Design review of the part built by this model. Coordinates are the model's own, in mm. Coordinates: 2 decimals unless noted, no trailing zeros. Order: outer loops, then holes, each group sorted by start corner. A loop starts at its lowest first (then second) coordinate and runs counter-clockwise, first axis right, second up. Notation, with made-up numbers: M 48,-9 L 69,-9 A23 cw 69,8 Z; hole C 27.25,53.25 d10. An arc over 180 degrees is marked long. Answer in a Markdown table with one row per item.
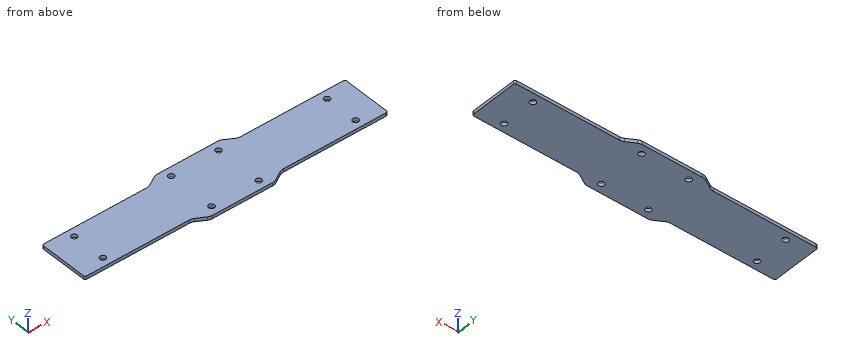
Autodesk Inventor part; units mm, degrees
ref_plane "YZ Plane" through (0, 0, 0) normal (1, 0, 0) x (0, 1, 0)
ref_plane "XZ Plane" through (0, 0, 0) normal (0, 1, 0) x (-1, 0, 0)
ref_plane "XY Plane" through (0, 0, 0) normal (0, 0, 1) x (1, 0, 0)
sketch "スケッチ1" plane through (0, 0, 0) normal (0, 0, 1) x (1, 0, 0)
  line L0 (-90.5, -15) -> (90.5, -15)
  line L1 (90.5, -15) -> (90.5, 15)
  line L2 (90.5, 15) -> (-90.5, 15)
  line L3 (-90.5, 15) -> (-90.5, -15)
  line L4 (-90.5, -15) -> (90.5, 15) construction
  line L5 (90.5, -15) -> (-90.5, 15) construction
  line L6 (-19.3, -19.3) -> (19.3, -19.3)
  line L7 (19.3, -19.3) -> (19.3, 19.3)
  line L8 (19.3, 19.3) -> (-19.3, 19.3)
  line L9 (-19.3, 19.3) -> (-19.3, -19.3)
  line L10 (-19.3, -19.3) -> (19.3, 19.3) construction
  line L11 (19.3, -19.3) -> (-19.3, 19.3) construction
  line L12 (-19.3, 19.3) -> (-26.7478, 15)
  line L13 (-19.3, -19.3) -> (-26.7478, -15)
  line L14 (19.3, -19.3) -> (26.7478, -15)
  line L15 (26.7478, 15) -> (19.3, 19.3)
  point P0 (0, 0)
  dimension "d0" = 181
  dimension "d1" = 30
  dimension "d2" = 38.6
  dimension "d3" = 38.6
  dimension "d4" = 150
  dimension "d5" = 150
extrude "プレート1" add sketch "スケッチ1" along normal blind 2
sketch "スケッチ2" plane through (0, 0, 2) normal (0, 0, 1) x (1, 0, 0)
  line L0 (-75.5, -10) -> (75.5, -10) construction
  line L1 (75.5, -10) -> (75.5, 10) construction
  line L2 (75.5, 10) -> (-75.5, 10) construction
  line L3 (-75.5, 10) -> (-75.5, -10) construction
  line L4 (-75.5, -10) -> (75.5, 10) construction
  line L5 (75.5, -10) -> (-75.5, 10) construction
  point P0 (0, 0)
  dimension "d7" = 151
  dimension "d8" = 20
hole "穴1" at (-75.5, 10, 2) at (-75.5, -10, 2) at (75.5, -10, 2) at (75.5, 10, 2) direction (0, 0, -1) diameter 3.5 depth 2 tip angle 118
sketch "スケッチ3" plane through (0, 0, 2) normal (0, 0, 1) x (1, 0, 0)
  line L0 (-14.1, -14.1) -> (14.1, -14.1) construction
  line L1 (14.1, -14.1) -> (14.1, 14.1) construction
  line L2 (14.1, 14.1) -> (-14.1, 14.1) construction
  line L3 (-14.1, 14.1) -> (-14.1, -14.1) construction
  line L4 (-14.1, -14.1) -> (14.1, 14.1) construction
  line L5 (14.1, -14.1) -> (-14.1, 14.1) construction
  point P0 (0, 0)
  dimension "d16" = 28.2
  dimension "d17" = 28.2
hole "穴2" at (14.1, 14.1, 2) at (14.1, -14.1, 2) at (-14.1, -14.1, 2) at (-14.1, 14.1, 2) direction (0, 0, -1) diameter 3.5 depth 2 tip angle 118
fillet "フィレット1" radius 5 8 edges at (26.7478, 15, 1) (19.3, 19.3, 1) (26.7478, -15, 1) (19.3, -19.3, 1) (-19.3, -19.3, 1) (-26.7478, -15, 1) (-26.7478, 15, 1) (-19.3, 19.3, 1)
fillet "フィレット2" radius 1 4 edges at (-90.5, 15, 1) (-90.5, -15, 1) (90.5, -15, 1) (90.5, 15, 1)
equation "\"d3\" = d2"
equation "\"d5\" = d4"
equation "\"d14\" = Thickness"
equation "\"d23\" = Thickness"
equation "\"d6\" = Thickness"
equation "\"BendRadius\" = Thickness"
equation "\"BendReliefWidth\" = Thickness"
equation "\"BendReliefDepth\" = 0.5 * Thickness"
equation "\"CornerReliefSize\" = 4 * Thickness"
equation "\"MinimumRemnant\" = 2 * Thickness"
equation "\"TransitionRadius\" = BendRadius"
equation "\"JacobiRadiusSize\" = BendRadius"
equation "\"GapSize\" = Thickness"
properties part number "T2.0_frame-base4"
(1) Add section B-B, the plane z = 1.7. Give the number of separate pieces and of enclosed holes in the cut face, and give its area (3 significant figures).
Return value:
| item | result |
|---|---|
| separate pieces | 1 |
| enclosed holes | 8 |
| area | 5,750 mm2 |
(2) Add section A-A, the plane x = -14.1. Give the boundary of the cut face in (y, z).
Return value:
| item | result |
|---|---|
| outline | M -19.3,0 L -15.85,0 L -15.85,2 L -19.3,2 Z; M -12.35,0 L 12.35,0 L 12.35,2 L -12.35,2 Z; M 15.85,0 L 19.3,0 L 19.3,2 L 15.85,2 Z |
(3) For line 1 along Y through (x, z) = (-14.1, 0.75); line 2 along X through (y, z) = (-14.1, 0.55); line 3 along X through (y, z) = (10, 1.1), list the stretches that pass through material, from the lowest coordinate up. Write a range as from..to.
Return value:
| item | result |
|---|---|
| line 1 | y = -19.3..-15.85, -12.35..12.35, 15.85..19.3 |
| line 2 | x = -90.49..-15.85, -12.35..12.35, 15.85..90.49 |
| line 3 | x = -90.5..-77.25, -73.75..73.75, 77.25..90.5 |
(4) Insertion check: pin 1 Ø5.5 at (x, y) = (14.1, 14.1) entering from +Z; pin 2 Ø3 at (x, y) = (-75.5, -10) entering from -Z; pin 3 Ø1 at (x, z) = (73, 1) entering from +Y; pin 4 Ø1 at (x, z) = (-49.5, 1.5) entering from -Y. Each pin has a flat end and moves straight along its axis. Give the tip position at first contact, or say it passes through.
Return value:
| item | result |
|---|---|
| pin 1 | stops at z = 2 |
| pin 2 | passes through |
| pin 3 | stops at y = 15 |
| pin 4 | stops at y = -15 |
(5) Add section D-D, the plane x = 70. Give the boundary of the cut face in (y, z).
Return value:
| item | result |
|---|---|
| outline | M -15,0 L 15,0 L 15,2 L -15,2 Z |
(6) Add section C-C, the plane y = 10. Give the boundary of the cut face in (x, z), and give its area (3 significant figures).
Return value:
| item | result |
|---|---|
| outline | M -90.5,0 L -77.25,0 L -77.25,2 L -90.5,2 Z; M -73.75,0 L 73.75,0 L 73.75,2 L -73.75,2 Z; M 77.25,0 L 90.5,0 L 90.5,2 L 77.25,2 Z |
| area | 348 mm2 |
